The model under review builds one solid part; all positions refer to its coordinate system, in mm. A direction names the side the tool comes from. Round coordinates to 2 decimals unless told otherwise and drop trailing zeros. Write each loop counter-clockwise with the first axis right and the second up, starting at its lowest first coordinate (ties: lowest second). Pieces come first, ordered by that corner, then holes. Notation, with made-up numbers: (-15.75, 76) - (-8.75, 76) arc R23 cw to (-8.75, 108) - close; hole circle Ø5 at (32.5, 83.5). An arc over 180 degrees is marked (long way). Write each question's results on one line, items separated by ' | '.
```python
from build123d import *
from build123d.topology import SkipClean

# Parameters (mm, degrees)
BOSS_EXTRUDE1_DEPTH                                 = 221.5
CSK_FOR_M3_COUNTERSUNK_FLAT_HEAD_SCREW1_D           = 3
CSK_FOR_M3_COUNTERSUNK_FLAT_HEAD_SCREW1_CSINK_D     = 5.5
CSK_FOR_M3_COUNTERSUNK_FLAT_HEAD_SCREW1_CSINK_ANGLE = 90
CSK_FOR_M3_COUNTERSUNK_FLAT_HEAD_SCREW4_D           = 3
CSK_FOR_M3_COUNTERSUNK_FLAT_HEAD_SCREW4_CSINK_D     = 5.5
CSK_FOR_M3_COUNTERSUNK_FLAT_HEAD_SCREW4_CSINK_ANGLE = 90
SKETCH12_W                                          = 8
SKETCH12_H                                          = 7
BOSS_EXTRUDE2_DEPTH                                 = 5.5
CUT_EXTRUDE1_DEPTH                                  = 359
BOSS_EXTRUDE3_DEPTH                                 = 3
BOSS_EXTRUDE4_DEPTH                                 = 2.5
BOSS_EXTRUDE4_DEPTH_BACK                            = 6
SKETCH19_W                                          = 0.6
SKETCH19_H                                          = 227
CUT_EXTRUDE2_DEPTH                                  = 10
SKETCH20_W                                          = 15.604741464
SKETCH20_H                                          = 2
CUT_EXTRUDE3_DEPTH                                  = 10
SKETCH21_W                                          = 0.6
SKETCH21_H                                          = 225
CUT_EXTRUDE4_DEPTH                                  = 10
SKETCH22_W                                          = 8.4
SKETCH22_H                                          = 5.5
CUT_EXTRUDE5_DEPTH                                  = 10
BOSS_EXTRUDE5_DEPTH                                 = 2
TAP_DRILL_FOR_M4X0_7_TAP1_D                         = 4
TAP_DRILL_FOR_M4X0_7_TAP1_DEPTH                     = 5
BOSS_EXTRUDE6_DEPTH                                 = 221.5
FILLET1_R                                           = 1
SKETCH30_R                                          = 2
BOSS_EXTRUDE7_DEPTH                                 = 4.5
BOSS_EXTRUDE8_DEPTH                                 = 1


with BuildPart() as part:
    # Sketch1 → Boss-Extrude1 (new body)
    with BuildSketch(Plane(origin=(0, 0, 0), x_dir=(1, 0, 0), z_dir=(0, 1, 0))):
        Polygon((0, 0), (0, 9), (9, 9), (9, 7), (2, 7), (2, 0), align=None)
    extrude(amount=BOSS_EXTRUDE1_DEPTH)

    # CSK for M3 Countersunk Flat Head Screw1 (through all)
    with Locations(Plane.ZY):
        with Locations((-4, 120)):
            CounterSinkHole(CSK_FOR_M3_COUNTERSUNK_FLAT_HEAD_SCREW1_D / 2, CSK_FOR_M3_COUNTERSUNK_FLAT_HEAD_SCREW1_CSINK_D / 2, counter_sink_angle=CSK_FOR_M3_COUNTERSUNK_FLAT_HEAD_SCREW1_CSINK_ANGLE)

    # CSK for M3 Countersunk Flat Head Screw4 (through all)
    with Locations(Plane(origin=(0, 0, -9), x_dir=(-1, 0, 0), z_dir=(0, 0, -1))):
        with Locations((-5, 40.25), (-5, 211)):
            CounterSinkHole(CSK_FOR_M3_COUNTERSUNK_FLAT_HEAD_SCREW4_D / 2, CSK_FOR_M3_COUNTERSUNK_FLAT_HEAD_SCREW4_CSINK_D / 2, counter_sink_angle=CSK_FOR_M3_COUNTERSUNK_FLAT_HEAD_SCREW4_CSINK_ANGLE)

    # Sketch12 → Boss-Extrude2 (add)
    with BuildSketch(Plane.XZ):
        with Locations((5, -3.5)):
            Rectangle(SKETCH12_W, SKETCH12_H)
    extrude(amount=-BOSS_EXTRUDE2_DEPTH)

    # Sketch13 → Cut-Extrude1 (cut)
    with BuildSketch(Plane(origin=(0, 221.5, 0), x_dir=(1, 0, 0), z_dir=(0, 1, 0))):
        Polygon((0, 8), (1, 9), (0, 9), align=None)
    extrude(amount=-CUT_EXTRUDE1_DEPTH, mode=Mode.SUBTRACT)

    # Sketch14 → Boss-Extrude3 (add)
    with BuildSketch(Plane.XZ):
        Polygon((0, 0), (9, 0), (9, -9), (1, -9), (0, -8), align=None)
    extrude(amount=BOSS_EXTRUDE3_DEPTH)

    # Sketch18 → Boss-Extrude4 (add, two sides: drawn at the far end of the back side and taken through both)
    with BuildSketch(Plane(origin=(0, 221.5, 0), x_dir=(1, 0, 0), z_dir=(0, 1, 0)).offset(-BOSS_EXTRUDE4_DEPTH_BACK)):
        Polygon((0, 0), (9, 0), (9, 9), (1, 9), (0, 8), align=None)
    extrude(amount=BOSS_EXTRUDE4_DEPTH + BOSS_EXTRUDE4_DEPTH_BACK)

    # Sketch19 → Cut-Extrude2 (cut)
    with BuildSketch(Plane.ZY):
        with Locations((-0.3, 110.5)):
            Rectangle(SKETCH19_W, SKETCH19_H)
    extrude(amount=-CUT_EXTRUDE2_DEPTH, mode=Mode.SUBTRACT)

    # Sketch20 → Cut-Extrude3 (cut)
    with BuildSketch(Plane.ZY):
        with Locations((-8.402370732, 223)):
            Rectangle(SKETCH20_W, SKETCH20_H)
    extrude(amount=-CUT_EXTRUDE3_DEPTH, mode=Mode.SUBTRACT)

    # Sketch21 → Cut-Extrude4 (cut)
    with BuildSketch(Plane(origin=(0, 0, -9), x_dir=(-1, 0, 0), z_dir=(0, 0, -1))):
        with Locations((-8.7, 109.5)):
            Rectangle(SKETCH21_W, SKETCH21_H)
    extrude(amount=-CUT_EXTRUDE4_DEPTH, mode=Mode.SUBTRACT)

    # Sketch22 → Cut-Extrude5 (cut)
    with BuildSketch(Plane(origin=(0, 0, -9), x_dir=(-1, 0, 0), z_dir=(0, 0, -1))):
        with Locations((-4.2, -0.25)):
            Rectangle(SKETCH22_W, SKETCH22_H)
    extrude(amount=-CUT_EXTRUDE5_DEPTH, mode=Mode.SUBTRACT)

    # Sketch26 → Boss-Extrude5 (add)
    with BuildSketch(Plane.XZ.offset(-2.5)):
        Polygon((8.4, -9), (8.4, -0.6), (0, -0.6), (0, -8), (1, -9), align=None)
    extrude(amount=BOSS_EXTRUDE5_DEPTH)

    # Tap Drill for M4x0.7 Tap1
    with Locations(Plane(origin=(0, 0.5, 0), x_dir=(-1, 0, 0), z_dir=(0, -1, 0))):
        with Locations((-5.4, 3.6)):
            Hole(TAP_DRILL_FOR_M4X0_7_TAP1_D / 2, depth=TAP_DRILL_FOR_M4X0_7_TAP1_DEPTH)

    # Sketch29 → Boss-Extrude6 (add)
    with BuildSketch(Plane(origin=(0, 222, 0), x_dir=(1, 0, 0), z_dir=(0, 1, 0))):
        Polygon((0, 8), (1, 9), (0, 9), align=None)
    extrude(amount=-BOSS_EXTRUDE6_DEPTH)

    # Fillet1
    fillet1_edges = [part.edges().sort_by_distance(p)[0] for p in [
        (0, 111.25, -9),
    ]]
    fillet(fillet1_edges, radius=FILLET1_R)

    # Sketch30 → Boss-Extrude7 (add)
    with SkipClean():  # the faces are left unmerged after this step: merging them gives an invalid solid
        with BuildSketch(Plane.XZ.offset(-0.5)):
            with BuildLine():
                Line((0, -0.6), (8.4, -0.6))
                Line((8.4, -0.6), (8.4, -9))
                Line((8.4, -9), (1, -9))
                ThreePointArc((1, -9), (0.292893219, -8.707106781), (0, -8))
                Line((0, -8), (0, -0.6))
            make_face()
            with Locations(Location((5.4, -3.6, 0), (0, 0, 270))):
                Circle(SKETCH30_R, mode=Mode.SUBTRACT)
        extrude(amount=BOSS_EXTRUDE7_DEPTH)
    add(part.part.scale(1), mode=Mode.REPLACE)  # the faces are merged on a copy

    # Sketch32 → Boss-Extrude8 (add)
    with SkipClean():  # the faces are left unmerged after this step: merging them gives an invalid solid
        with BuildSketch(Plane(origin=(0, 222, 0), x_dir=(1, 0, 0), z_dir=(0, 1, 0))):
            with BuildLine():
                Line((0, 0.6), (8.4, 0.6))
                Line((8.4, 0.6), (8.4, 9))
                Line((8.4, 9), (1, 9))
                ThreePointArc((1, 9), (0.292893219, 8.707106781), (0, 8))
                Line((0, 8), (0, 0.6))
            make_face()
        extrude(amount=BOSS_EXTRUDE8_DEPTH)


solid = part.part
```
Q1. For probe 1 along Y at (x, z) = (5, -7.5); probe 2 along Y at (x, z) = (1.65, -4); probe 3 along Y at (x, z) = (3.5, -1.5), list the stretches that pass through material, from the lowest coordinate up.
Evaluation:
probe 1: y = -4 to 38.75, 41.75 to 209.5, 212.5 to 223 | probe 2: y = -4 to 118.5, 121.5 to 223 | probe 3: y = -4 to 5.5, 215.5 to 223
Q2. Tool access review of faces 1 (the flat face through (5, 108, -9)), 2 (the flat face through (5, 215.5, -4)): name each direction out of +Z, -Z, +X, -X, +Y, -Y from which nothing blocks a thin tool from reaching the whole face with its end or side.
Evaluation:
face 1: -Z, +X, -X, +Y, -Y | face 2: +Z, +X
Q3. Insertion check: P1, Ø5, axis at y = 120, z = -4, coming from the +X side; P2, Ø1.8, axis at x = 5, y = 40.25, coming from the +Z side; P3, Ø1, axis at x = 6, y = 42, coming from the -Z side; P4, Ø3, axis at y = 26.5, z = -6, coming from the -X side. Each pin has a flat end and moves straight along its axis. Give the tip position at first contact, or say it passes through.
Evaluation:
P1: stops at x = 2 | P2: passes through | P3: stops at z = -8.77 | P4: stops at x = 0
Q4. We need section A-A (y = 65). State the section outline as (x, z) points.
Evaluation:
outline: (0, -8) arc R1 ccw to (1, -9) - (8.4, -9) - (8.4, -7) - (2, -7) - (2, -0.6) - (0, -0.6) - close
